Part model, mm, in its own coordinate system. A direction names the side the tool comes from. Give positions to 0.01 mm unless a question says otherwise; leave off trailing zeros. Write each loop counter-clockwise with the first axis right and the second up, starting at its lowest first coordinate (ties: lowest second). Pieces come first, ordered by that corner, then holes.
from build123d import *

# Parameters (mm, degrees)
SKETCH1_R           = 4.5000037
BOSS_EXTRUDE1_DEPTH = 3.75000012
BOSS_EXTRUDE2_START = 1.750000056
SKETCH2_R           = 4.5000037
SKETCH2_R_2         = 3.499999998
SKETCH2_R_3         = 1.25000004
BOSS_EXTRUDE2_DEPTH = 1.750000056
SKETCH4_R           = 2.75000466
SKETCH4_R_2         = 1.25000004
CUT_EXTRUDE1_DEPTH  = 0.875000028
SKETCH6_R           = 4.5000037
SKETCH6_R_2         = 3.5000057
CUT_EXTRUDE2_DEPTH  = 0.875000028
SKETCH10_R          = 0.62500002
SKETCH10_R_2        = 4.5000037
BOSS_EXTRUDE4_DEPTH = 1.750000056
CHAMFER2_SIZE       = 1.00000054
CHAMFER2_SIZE2      = 0.577350581


with BuildPart() as part:
    # Sketch1 → Boss-Extrude1 (new body)
    with BuildSketch(Plane.XY):
        with Locations((-10.24995918, 0)):
            Circle(SKETCH1_R)
        Polygon((-10.24995918, 2.999994), (-10.594624819, 2.728309468), (-10.996027349, 2.905743672), (-11.262299488, 2.55687975), (-11.695217312, 2.628914782), (-11.866365092, 2.224791874), (-12.303596391, 2.186901508), (-12.368865968, 1.752912142), (-12.782937891, 1.60747717), (-12.738228138, 1.170890494), (-13.103123023, 0.927049129), (-12.951243218, 0.515297489), (-13.244033377, 0.188371182), (-12.994526687, -0.172673551), (-13.196815038, -0.562142819), (-12.865358886, -0.849794878), (-12.964434908, -1.27733532), (-12.571855902, -1.473520467), (-12.561494285, -1.912268145), (-12.132459609, -2.004659346), (-12.01331141, -2.427046129), (-11.574778889, -2.409838105), (-11.354330629, -2.789323879), (-10.933854876, -2.663597874), (-10.625958129, -2.976338151), (-10.24995918, -2.749993992), (-9.873960231, -2.976338151), (-9.566063484, -2.663597874), (-9.145587731, -2.789323879), (-8.925139471, -2.409838105), (-8.48660695, -2.427046129), (-8.367458751, -2.004659346), (-7.938424075, -1.912268145), (-7.928062458, -1.473520467), (-7.535483452, -1.27733532), (-7.634559474, -0.849794878), (-7.303103322, -0.562142819), (-7.505391673, -0.172673551), (-7.255884983, 0.188371182), (-7.548675142, 0.515297489), (-7.396795337, 0.927049129), (-7.761690222, 1.170890494), (-7.716980469, 1.60747717), (-8.131052392, 1.752912142), (-8.196321969, 2.186901508), (-8.633553268, 2.224791874), (-8.804701048, 2.628914782), (-9.237618872, 2.55687975), (-9.503891011, 2.905743672), (-9.905293541, 2.728309468), align=None, mode=Mode.SUBTRACT)
    extrude(amount=-BOSS_EXTRUDE1_DEPTH)

    # Sketch2 → Boss-Extrude2 (add)
    # profile 1 of 2: a face of its own
    with BuildSketch(Plane.XY.offset(BOSS_EXTRUDE2_START)):
        with Locations((-10.24995918, 0)):
            Circle(SKETCH2_R)
        with Locations((-10.24995918, 0)):
            Circle(SKETCH2_R_2, mode=Mode.SUBTRACT)
    # profile 2 of 2: a face of its own
    with BuildSketch(Plane.XY.offset(BOSS_EXTRUDE2_START)):
        with Locations((-10.24995918, 0)):
            Circle(SKETCH2_R_2)
        with Locations((-10.24995918, 0)):
            Circle(SKETCH2_R_3, mode=Mode.SUBTRACT)
    extrude(amount=-BOSS_EXTRUDE2_DEPTH)

    # Sketch4 → Cut-Extrude1 (cut)
    with BuildSketch(Plane.XY.offset(1.750000056)):
        with Locations((-10.24995918, 0)):
            Circle(SKETCH4_R)
        with Locations((-10.24995918, 0)):
            Circle(SKETCH4_R_2, mode=Mode.SUBTRACT)
    extrude(amount=-CUT_EXTRUDE1_DEPTH, mode=Mode.SUBTRACT)

    # Sketch6 → Cut-Extrude2 (cut)
    with BuildSketch(Plane.XY.offset(1.750000056)):
        with Locations((-10.24995918, 0)):
            Circle(SKETCH6_R)
        with Locations((-10.24995918, 0)):
            Circle(SKETCH6_R_2, mode=Mode.SUBTRACT)
    extrude(amount=-CUT_EXTRUDE2_DEPTH, mode=Mode.SUBTRACT)

    # Sketch10 → Boss-Extrude4 (add)
    with BuildSketch(Plane.XY.offset(1.750000056)):
        with BuildLine():
            Line((-8.086927824, 17.701557226), (-6.029886341, 6.622035833))
            ThreePointArc((-6.029886341, 6.622035833), (-5.20161423, 5.04834495), (-3.627923347, 4.220072839))
            Line((-3.627923347, 4.220072839), (7.451598046, 2.163031356))
            ThreePointArc((7.451598046, 2.163031356), (9.25000182, 0), (7.451598046, -2.163031356))
            Line((7.451598046, -2.163031356), (-3.627923347, -4.220072839))
            ThreePointArc((-3.627923347, -4.220072839), (-5.20161423, -5.04834495), (-6.029886341, -6.622035833))
            Line((-6.029886341, -6.622035833), (-8.086927824, -17.701557226))
            ThreePointArc((-8.086927824, -17.701557226), (-10.24995918, -19.499961), (-12.412990536, -17.701557226))
            Line((-12.412990536, -17.701557226), (-14.470032019, -6.622035833))
            ThreePointArc((-14.470032019, -6.622035833), (-15.29830413, -5.04834495), (-16.871995013, -4.220072839))
            Line((-16.871995013, -4.220072839), (-27.951516406, -2.163031356))
            ThreePointArc((-27.951516406, -2.163031356), (-29.74992018, 0), (-27.951516406, 2.163031356))
            Line((-27.951516406, 2.163031356), (-16.871995013, 4.220072839))
            ThreePointArc((-16.871995013, 4.220072839), (-15.29830413, 5.04834495), (-14.470032019, 6.622035833))
            Line((-14.470032019, 6.622035833), (-12.412990536, 17.701557226))
            ThreePointArc((-12.412990536, 17.701557226), (-10.24995918, 19.499961), (-8.086927824, 17.701557226))
        make_face()
        with Locations((-10.24995918, 15.87496698)):
            Circle(SKETCH10_R, mode=Mode.SUBTRACT)
        with Locations((-10.24995918, 12.87497298)):
            Circle(SKETCH10_R, mode=Mode.SUBTRACT)
        with Locations((-10.24995918, 9.87497898)):
            Circle(SKETCH10_R, mode=Mode.SUBTRACT)
        with Locations((-10.24995918, 6.87498498)):
            Circle(SKETCH10_R, mode=Mode.SUBTRACT)
        with Locations((5.6250078, 0)):
            Circle(SKETCH10_R, mode=Mode.SUBTRACT)
        with Locations((2.6250138, 0)):
            Circle(SKETCH10_R, mode=Mode.SUBTRACT)
        with Locations((-0.3749802, 0)):
            Circle(SKETCH10_R, mode=Mode.SUBTRACT)
        with Locations((-3.3749742, 0)):
            Circle(SKETCH10_R, mode=Mode.SUBTRACT)
        with Locations((-10.24995918, -15.87496698)):
            Circle(SKETCH10_R, mode=Mode.SUBTRACT)
        with Locations((-10.24995918, -12.87497298)):
            Circle(SKETCH10_R, mode=Mode.SUBTRACT)
        with Locations((-10.24995918, -9.87497898)):
            Circle(SKETCH10_R, mode=Mode.SUBTRACT)
        with Locations((-10.24995918, -6.87498498)):
            Circle(SKETCH10_R, mode=Mode.SUBTRACT)
        with Locations((-26.12492616, 0)):
            Circle(SKETCH10_R, mode=Mode.SUBTRACT)
        with Locations((-23.12493216, 0)):
            Circle(SKETCH10_R, mode=Mode.SUBTRACT)
        with Locations((-20.12493816, 0)):
            Circle(SKETCH10_R, mode=Mode.SUBTRACT)
        with Locations((-17.12494416, 0)):
            Circle(SKETCH10_R, mode=Mode.SUBTRACT)
        with Locations((-10.24995918, 0)):
            Circle(SKETCH10_R_2, mode=Mode.SUBTRACT)
    extrude(amount=-BOSS_EXTRUDE4_DEPTH)

    # Chamfer2
    chamfer2_edges = [part.edges().sort_by_distance(p)[0] for p in [
        (-14.74996288, 0, 0),
    ]]
    chamfer2_side = [part.faces().sort_by_distance(p)[0] for p in [
        (-14.74996288, 0, -1.87500006),
    ]]
    chamfer(chamfer2_edges, length=CHAMFER2_SIZE, length2=CHAMFER2_SIZE2, reference=chamfer2_side[0])


solid = part.part
1) Flat gauge pins, fed straight in: P1, Ø0.8, axis at x = -10.25, y = -12.87, coming from the -Z side; P2, Ø1.6, axis at x = -10.25, y = 15.87, coming from the -Z side; P3, Ø3, axis at y = -12, z = 0, coming from the -X side. Where does each tip first touch, or does it go through?
Check result:
P1: passes through
P2: stops at z = 0
P3: stops at x = -13.75
2) Drill centre lines: L1, parallel to Y at x = -10, z = -0.9; L2, parallel to X at y = 9.5, z = 0.7; L3, parallel to Z at x = -9, y = 5.5. Where is each one in solid material? Low to high.
Check result:
L1: y = -4.55 to -2.9, 2.8 to 4.55
L2: x = -13.94 to -10.75, -9.75 to -6.56
L3: z = 0 to 1.75
3) 3-axis set-ups, long thin cutter, end or side, ignore diameter. For faces 1 (the cylindrical face through (-5.958, 1.352, -2.356)), 2 (the cylindrical face through (-10.874, 12.902, 0.887)): which of +Z, -Z, +X, -X, +Y, -Y reach the whole face in a straight line?
Check result:
face 1: -Z
face 2: +Z, -Z
4) Mould opens along X. For faces 3 (the cylindrical face through (-10.874, -12.847, 0.887)), 4 (the flat face through (-22.489, 3.177, 0.887)), 5 (the cylindrical face through (-10.746, -10.255, 0.887)), 6 (the flat face through (-7.073, 12.239, 0.887)) say: +X half, -X half, draft (parallel to the pull), parting line (faces both ways), or undercut.
Check result:
face 3: undercut
face 4: -X half
face 5: undercut
face 6: +X half
5) Saw through at A-A (x = 5.5). Write the cut outline in (y, z), and give its area (3 significant figures).
Check result:
outline: (-2.53, 0) - (-0.61, 0) - (-0.61, 1.75) - (-2.53, 1.75) - close; (0.61, 0) - (2.53, 0) - (2.53, 1.75) - (0.61, 1.75) - close
area: 6.70 mm2
6) Saw through at B-B (x = -18.5). Write the cut outline in (y, z), and give its area (3 significant figures).
Check result:
outline: (-3.92, 0) - (3.92, 0) - (3.92, 1.75) - (-3.92, 1.75) - close
area: 13.7 mm2
